```python
from build123d import *

# Parameters (mm, degrees)
F0_W     = 460
F0_H     = 38
F1_DEPTH = 3
F2_W     = 27
F2_H     = 3
F2_W_2   = 92
F3_DEPTH = 3
F5_DEPTH = 3
F6_W     = 3
F6_H     = 8
F7_DEPTH = 3
F9_DEPTH = 3
F11_D    = 3


with BuildPart() as f1:
    # F0 (on Front) → F1 (new body)
    with BuildSketch(Plane.XZ):
        Polygon((-343.484793, -216.105753), (-316.484793, -216.105753), (-316.484793, -106.105753), (-343.484793, -106.105753), (-343.484793, -121.105753), (-346.484793, -121.105753), (-346.484793, -106.105753), (-806.484793, -106.105753), (-806.484793, -121.105753), (-809.484793, -121.105753), (-809.484793, -106.105753), (-836.484793, -106.105753), (-836.484793, -216.105753), (-809.484793, -216.105753), (-809.484793, -201.105753), (-806.484793, -201.105753), (-806.484793, -216.105753), (-346.484793, -216.105753), (-346.484793, -201.105753), (-343.484793, -201.105753), align=None)
        with Locations((-576.484793, -165.105753)):
            Rectangle(F0_W, F0_H, mode=Mode.SUBTRACT)
    extrude(amount=F1_DEPTH)

    # F2 (on face) → F3 (join)
    with BuildSketch(Plane.XZ.offset(3)):
        with Locations((-822.984793, -104.605753)):
            Rectangle(F2_W, F2_H)
        with Locations((-329.984793, -104.605753)):
            Rectangle(F2_W, F2_H)
        with Locations((-671.484793, -104.605753)):
            Rectangle(F2_W_2, F2_H)
        with Locations((-481.484793, -104.605753)):
            Rectangle(F2_W_2, F2_H)
    extrude(amount=-F3_DEPTH)

    # F4 (on face) → F5 (cut, through all)
    with BuildSketch(Plane.XZ.offset(3)):
        with BuildLine():
            Line((-377.784793, -206.105753), (-377.784793, -196.105753))
            ThreePointArc((-377.784793, -196.105753), (-383.034793, -190.855753), (-388.284793, -196.105753))
            Line((-388.284793, -196.105753), (-388.284793, -206.105753))
            ThreePointArc((-388.284793, -206.105753), (-383.034793, -211.355753), (-377.784793, -206.105753))
        make_face()
        with BuildLine():
            Line((-764.684793, -206.105753), (-764.684793, -196.105753))
            ThreePointArc((-764.684793, -196.105753), (-769.934793, -190.855753), (-775.184793, -196.105753))
            Line((-775.184793, -196.105753), (-775.184793, -206.105753))
            ThreePointArc((-775.184793, -206.105753), (-769.934793, -211.355753), (-764.684793, -206.105753))
        make_face()
    extrude(amount=-F5_DEPTH, mode=Mode.SUBTRACT)

    # F6 (on face) → F7 (cut)
    with BuildSketch(Plane.XZ.offset(3)):
        with Locations((-726.484793, -212.105753)):
            Rectangle(F6_W, F6_H)
        with Locations((-726.484793, -188.105753)):
            Rectangle(F6_W, F6_H)
        with Locations((-626.484793, -188.105753)):
            Rectangle(F6_W, F6_H)
        with Locations((-626.484793, -212.105753)):
            Rectangle(F6_W, F6_H)
        with Locations((-526.484793, -188.105753)):
            Rectangle(F6_W, F6_H)
        with Locations((-526.484793, -212.105753)):
            Rectangle(F6_W, F6_H)
        with Locations((-426.484793, -188.105753)):
            Rectangle(F6_W, F6_H)
        with Locations((-426.484793, -212.105753)):
            Rectangle(F6_W, F6_H)
    extrude(amount=-F7_DEPTH, mode=Mode.SUBTRACT)

    # F8 (on face) → F9 (join)
    with BuildSketch(Plane.XZ.offset(3)):
        with BuildLine():
            Line((-760.769642, -216.105753), (-779.099944, -216.105753))
            ThreePointArc((-779.099944, -216.105753), (-769.934793, -220.105753), (-760.769642, -216.105753))
        make_face()
        with BuildLine():
            Line((-373.869642, -216.105753), (-392.199944, -216.105753))
            ThreePointArc((-392.199944, -216.105753), (-383.034793, -220.105753), (-373.869642, -216.105753))
        make_face()
    extrude(amount=-F9_DEPTH)

    # F11 (through all)
    with Locations(Plane(origin=(0, 0, 0), x_dir=(-1, 0, 0), z_dir=(0, 1, 0))):
        with Locations((329.984793, -113.105753)):
            Hole(F11_D / 2)


solid = f1.part
```
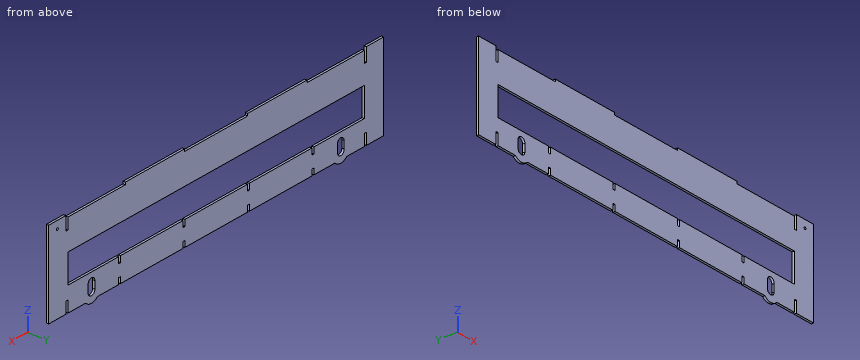
Build history of the part. All positions in model axes, mm. Round coordinates to 2 decimals unless told otherwise and drop trailing zeros. Loops run counter-clockwise (first coordinate to the right, second up) from the corner with the lowest first, then second, coordinate; pieces in that order, holes last. Notation, with made-up numbers: M 62,-31.75 L 94,-31.75 A21 cw 94,4.25 Z; hole C 32.25,44 d5. An arc over 180 degrees is marked long. Answer as CSV lines item,"result".
1. Wall check: probe 1 along X at (y, z) = (-2.75, -205.5); probe 2 along X at (y, z) = (-0.3, -151.5); probe 3 along Z at (x, y) = (-722, -1.9). Give the ranges that are in metal, low to high. Write a range as [from, to].
Resolved:
probe 1,"x = [-836.48, -809.48], [-806.48, -775.18], [-764.68, -388.28], [-377.78, -346.48], [-343.48, -316.48]"
probe 2,"x = [-836.48, -806.48], [-346.48, -316.48]"
probe 3,"z = [-216.11, -184.11], [-146.11, -106.11]"
2. Cut at A-A on z = -155.5. Write the cut outline in (x, y).
Resolved:
outline,"M -836.48,-3 L -806.48,-3 L -806.48,0 L -836.48,0 Z; M -346.48,-3 L -316.48,-3 L -316.48,0 L -346.48,0 Z"
3. Cut at C-C on y = -2.05. Count the separate pieces of the cut face and the enclosed holes in it, then the cut area to 3 significant figures.
Resolved:
separate pieces,"1"
enclosed holes,"4"
area,"39,800 mm²"
4. Cut at B-B on x = -677. Write the cut outline in (y, z).
Resolved:
outline,"M -3,-216.11 L 0,-216.11 L 0,-184.11 L -3,-184.11 Z; M -3,-146.11 L 0,-146.11 L 0,-103.11 L -3,-103.11 Z"
5. Flat gauge pins, fed straight in: P1, Ø8, axis at x = -426.5, z = -140.5, coming from the +Y side; P2, Ø0.9, axis at x = -381, y = -1, coming from the +Z side. Where does each tip first touch, or does it go through?
Resolved:
P1,"stops at y = 0"
P2,"stops at z = -106.11"
